Here's the drawing with two shaded views (mm, measured from the low corner). I have some questions. A direction names the side the tool comes from. Coordinates: 2 decimals unless noted, no trailing zeros. Loops run counter-clockwise (first coordinate to the right, second up) from the corner with the lowest first, then second, coordinate; pieces in that order, holes last. Notation, with made-up numbers: (-33, -5.5) - (2, -5.5) arc R21 cw to (2, 10.5) - close; hole circle Ø9 at (22, 50). An arc over 180 degrees is marked (long way). Use a Markdown table: item, result.
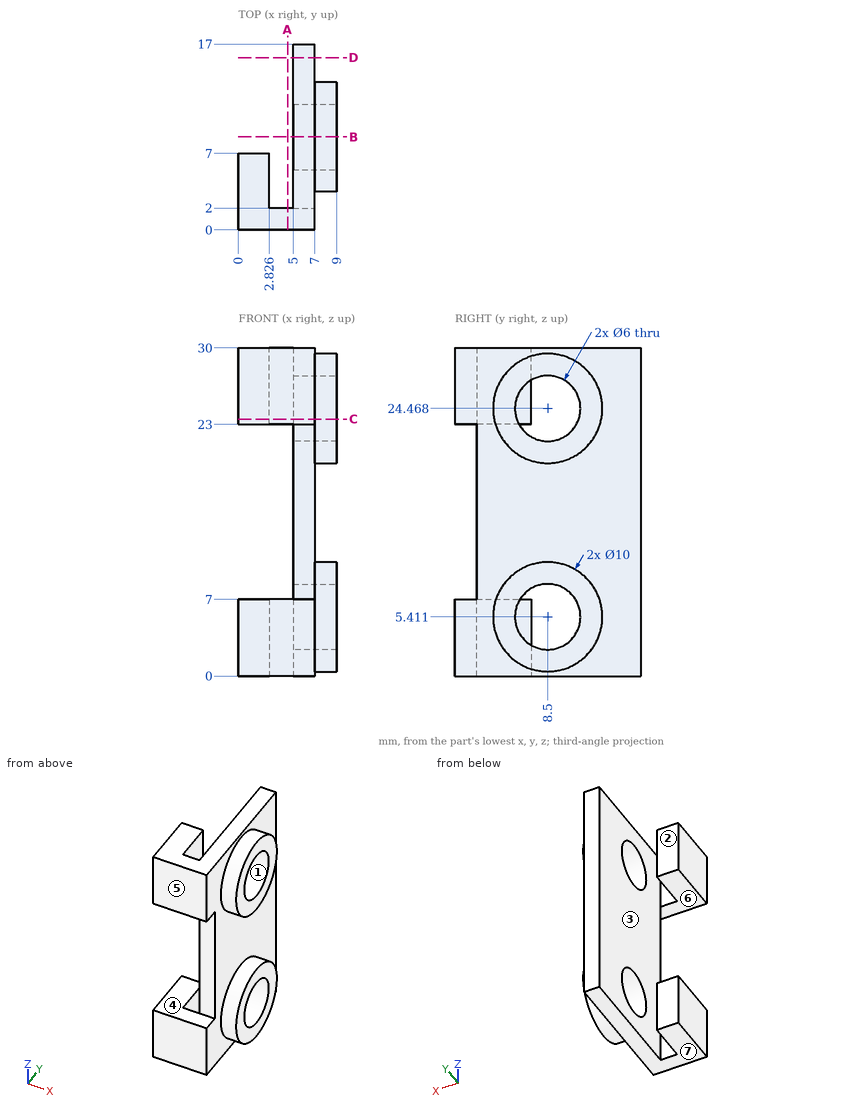
Q1. Will these pins go through, and if not, where does the flat tip stop? P1, Ø5, axis at y = 8.5, z = 24.47, coming from the +X side; P2, Ø5, axis at y = 14.5, z = 22, coming from the -X side; P3, Ø0.7, axis at x = 3.5, z = 25.5, coming from the +Y side; P4, Ø2, axis at x = 4.5, y = 4, coming from the -Z side.
Check values:
| item | result |
|---|---|
| P1 | x = 2.83 |
| P2 | x = 5 |
| P3 | y = 2 |
| P4 | z = 0 |
Q2. I want a section at B-B, the plane y = 8.5. Write out the boundary of the cut face in (x, z).
Check values:
| item | result |
|---|---|
| outline | (5, 0) - (7, 0) - (7, 0.41) - (9, 0.41) - (9, 2.41) - (5, 2.41) - close; (5, 8.41) - (9, 8.41) - (9, 10.41) - (7, 10.41) - (7, 19.47) - (9, 19.47) - (9, 21.47) - (5, 21.47) - close; (5, 27.47) - (9, 27.47) - (9, 29.47) - (7, 29.47) - (7, 30) - (5, 30) - close |
Q3. Please list where these lines run through material, in increasing order: L1, parallel to Z at x = 5.75, y = 1.25; L2, parallel to X at y = 8, z = 17.75; L3, parallel to X at y = 11, z = 8.25. Write a range as from..to.
Check values:
| item | result |
|---|---|
| L1 | 0..7, 23..30 |
| L2 | 5..7 |
| L3 | 5..9 |
Q4. I want a section at D-D, the plane y = 15.75. Write out the boundary of the cut face in (x, z), then the cut area to 3 significant figures.
Check values:
| item | result |
|---|---|
| outline | (5, 0) - (7, 0) - (7, 30) - (5, 30) - close |
| area | 60.0 mm^2 |
Q5. If we mould it in two halves opening along Z, with no side actions, what happens to the marked faces 4, 5, 6 and 7? For each: pulls with the +Z half, pulls with the -Z half, needs draft (parallel to the pull), parting line crosses it, or undercut.
Check values:
| item | result |
|---|---|
| face 4 | undercut |
| face 5 | needs draft |
| face 6 | undercut |
| face 7 | pulls with the -Z half |
Q6. I want a section at C-C, the plane z = 23.5. Write out the boundary of the cut face in (x, y) (1 decimal).
Check values:
| item | result |
|---|---|
| outline | (0, 0) - (7, 0) - (7, 3.6) - (9, 3.6) - (9, 5.7) - (5, 5.7) - (5, 2) - (2.8, 2) - (2.8, 7) - (0, 7) - close; (5, 11.3) - (9, 11.3) - (9, 13.4) - (7, 13.4) - (7, 17) - (5, 17) - close |
Q7. Which directions (+Z, -Z, +X, -X, +Y, -Y) give clear straight access to the entire face, cutting with the end or side of a thin tool? Please do the marked faces 1, 2 and 3.
Check values:
| item | result |
|---|---|
| face 1 | +X |
| face 2 | +Z, -Z, -X, +Y |
| face 3 | +Z, -Z, +Y |
Q8. I want a section at A-A, the plane x = 4.5. Write out the boundary of the cut face in (y, z).
Check values:
| item | result |
|---|---|
| outline | (0, 0) - (2, 0) - (2, 7) - (0, 7) - close; (0, 23) - (2, 23) - (2, 30) - (0, 30) - close |
